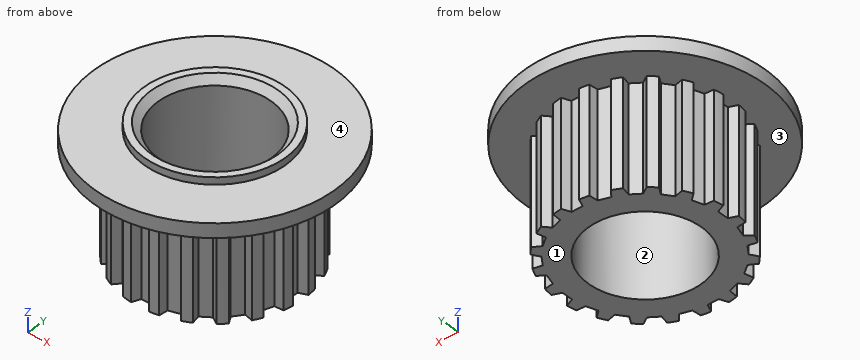
```python
from build123d import *

# Parameters (mm, degrees)
CUT_EXTRUDE1_DEPTH       = 3
CHAMFER1_SIZE            = 0.259911356
CHAMFER1_SIZE2           = 0.226339217
CUT_EXTRUDE2_START       = 1
CUT_EXTRUDE2_2_OUTLINE_W = 16
CUT_EXTRUDE2_2_OUTLINE_H = 4
CUT_EXTRUDE2_2_DEPTH     = 6.45
CUT_EXTRUDE2_START_2     = 7.45
CUT_EXTRUDE2_3_OUTLINE_R = 5
CUT_EXTRUDE2_3_DEPTH     = 7.5


with BuildPart() as part:
    # Sketch1 → Revolve1 (revolve)
    with BuildSketch(Plane.XY.offset(3.725), mode=Mode.PRIVATE) as revolve1_sk:
        Polygon((1.614337285, 9), (0, 9), (0, 5), (0.595828025, 5), (1.614337285, 5.592863599), align=None)
    revolve(revolve1_sk.sketch.rotate(Axis((0, 9, 3.725), (0, -1, 0)), 270), axis=Axis((0, 9, 3.725), (0, -1, 0)))

    # Sketch2 → Cut-Extrude1 (cut)
    with BuildSketch(Plane(origin=(0, 9, 0), x_dir=(-1, 0, 0), z_dir=(0, 1, 0))):
        Polygon((0.877701457, 2.974684409), (1.088643091, 4.109953963), (0.210941634, 4.860269554), (-0.877701457, 4.475315591), (-1.088643091, 3.340046037), (-0.210941634, 2.589730446), align=None)
    extrude(amount=-CUT_EXTRUDE1_DEPTH, mode=Mode.SUBTRACT)

    # Chamfer1
    chamfer1_edges = [part.edges().sort_by_distance(p)[0] for p in [
        (0, 9, 5.339337285),
    ]]
    chamfer1_side = [part.faces().sort_by_distance(p)[0] for p in [
        (0, 9, 5.293676931),
    ]]
    chamfer(chamfer1_edges, length=CHAMFER1_SIZE, length2=CHAMFER1_SIZE2, reference=chamfer1_side[0])

    # Cut-Extrude2 2 outline → Cut-Extrude2 2 (cut)
    with BuildSketch(Plane.XY.offset(CUT_EXTRUDE2_START)):
        with Locations((0, 7)):
            Rectangle(CUT_EXTRUDE2_2_OUTLINE_W, CUT_EXTRUDE2_2_OUTLINE_H)
    extrude(amount=CUT_EXTRUDE2_2_DEPTH, mode=Mode.SUBTRACT)


with BuildPart() as body_2:
    # Cut-Extrude2: read off the stored shape, not the designer's step
    # Cut-Extrude2 outline → Cut-Extrude2 (revolve)
    with BuildSketch(Plane.XZ):
        Polygon((4, 7.45), (5, 7.45), (5, 14.95), (8.5, 14.95), (8.5, 15.95), (5, 15.95), (5, 16.45), (4.5, 16.45), (4, 15.95), align=None)
    revolve(axis=Axis((0, 0, 0), (0, 0, 1)))

    # Cut-Extrude2 3 outline → Cut-Extrude2 3 (add)
    with BuildSketch(Plane.XY.offset(CUT_EXTRUDE2_START_2)):
        with BuildLine():
            Line((1.30065941, -6.077376909), (1.350072562, -5.449523289))
            Line((1.350072562, -5.449523289), (2.110917775, -5.202309694))
            Line((2.110917775, -5.202309694), (2.519936953, -5.681209621))
            ThreePointArc((2.519936953, -5.681209621), (2.821550956, -5.537605548), (3.115013354, -5.37800305))
            Line((3.115013354, -5.37800305), (2.967990615, -4.765609269))
            Line((2.967990615, -4.765609269), (3.615204211, -4.295381068))
            Line((3.615204211, -4.295381068), (4.152192781, -4.624448087))
            ThreePointArc((4.152192781, -4.624448087), (4.394668645, -4.394668645), (4.624448087, -4.152192781))
            Line((4.624448087, -4.152192781), (4.295381068, -3.615204211))
            Line((4.295381068, -3.615204211), (4.765609269, -2.967990615))
            Line((4.765609269, -2.967990615), (5.37800305, -3.115013354))
            ThreePointArc((5.37800305, -3.115013354), (5.537605548, -2.821550956), (5.681209621, -2.519936953))
            Line((5.681209621, -2.519936953), (5.202309694, -2.110917775))
            Line((5.202309694, -2.110917775), (5.449523289, -1.350072562))
            Line((5.449523289, -1.350072562), (6.077376909, -1.30065941))
            ThreePointArc((6.077376909, -1.30065941), (6.138483037, -0.9722402), (6.181854773, -0.641012138))
            Line((6.181854773, -0.641012138), (5.6, -0.4))
            Line((5.6, -0.4), (5.6, 0.4))
            Line((5.6, 0.4), (6.181854773, 0.641012138))
            ThreePointArc((6.181854773, 0.641012138), (6.138483037, 0.9722402), (6.077376909, 1.30065941))
            Line((6.077376909, 1.30065941), (5.449523289, 1.350072562))
            Line((5.449523289, 1.350072562), (5.202309694, 2.110917775))
            Line((5.202309694, 2.110917775), (5.681209621, 2.519936953))
            ThreePointArc((5.681209621, 2.519936953), (5.537605548, 2.821550956), (5.37800305, 3.115013354))
            Line((5.37800305, 3.115013354), (4.765609269, 2.967990615))
            Line((4.765609269, 2.967990615), (4.295381068, 3.615204211))
            Line((4.295381068, 3.615204211), (4.624448087, 4.152192781))
            ThreePointArc((4.624448087, 4.152192781), (4.394668645, 4.394668645), (4.152192781, 4.624448087))
            Line((4.152192781, 4.624448087), (3.615204211, 4.295381068))
            Line((3.615204211, 4.295381068), (2.967990615, 4.765609269))
            Line((2.967990615, 4.765609269), (3.115013354, 5.37800305))
            ThreePointArc((3.115013354, 5.37800305), (2.821550956, 5.537605548), (2.519936953, 5.681209621))
            Line((2.519936953, 5.681209621), (2.110917775, 5.202309694))
            Line((2.110917775, 5.202309694), (1.350072562, 5.449523289))
            Line((1.350072562, 5.449523289), (1.30065941, 6.077376909))
            ThreePointArc((1.30065941, 6.077376909), (0.9722402, 6.138483037), (0.641012138, 6.181854773))
            Line((0.641012138, 6.181854773), (0.4, 5.6))
            Line((0.4, 5.6), (-0.4, 5.6))
            Line((-0.4, 5.6), (-0.641012138, 6.181854773))
            ThreePointArc((-0.641012138, 6.181854773), (-0.9722402, 6.138483037), (-1.30065941, 6.077376909))
            Line((-1.30065941, 6.077376909), (-1.350072562, 5.449523289))
            Line((-1.350072562, 5.449523289), (-2.110917775, 5.202309694))
            Line((-2.110917775, 5.202309694), (-2.519936953, 5.681209621))
            ThreePointArc((-2.519936953, 5.681209621), (-2.821550956, 5.537605548), (-3.115013354, 5.37800305))
            Line((-3.115013354, 5.37800305), (-2.967990615, 4.765609269))
            Line((-2.967990615, 4.765609269), (-3.615204211, 4.295381068))
            Line((-3.615204211, 4.295381068), (-4.152192781, 4.624448087))
            ThreePointArc((-4.152192781, 4.624448087), (-4.394668645, 4.394668645), (-4.624448087, 4.152192781))
            Line((-4.624448087, 4.152192781), (-4.295381068, 3.615204211))
            Line((-4.295381068, 3.615204211), (-4.765609269, 2.967990615))
            Line((-4.765609269, 2.967990615), (-5.37800305, 3.115013354))
            ThreePointArc((-5.37800305, 3.115013354), (-5.537605548, 2.821550956), (-5.681209621, 2.519936953))
            Line((-5.681209621, 2.519936953), (-5.202309694, 2.110917775))
            Line((-5.202309694, 2.110917775), (-5.449523289, 1.350072562))
            Line((-5.449523289, 1.350072562), (-6.077376909, 1.30065941))
            ThreePointArc((-6.077376909, 1.30065941), (-6.138483037, 0.9722402), (-6.181854773, 0.641012138))
            Line((-6.181854773, 0.641012138), (-5.6, 0.4))
            Line((-5.6, 0.4), (-5.6, -0.4))
            Line((-5.6, -0.4), (-6.181854773, -0.641012138))
            ThreePointArc((-6.181854773, -0.641012138), (-6.138483037, -0.9722402), (-6.077376909, -1.30065941))
            Line((-6.077376909, -1.30065941), (-5.449523289, -1.350072562))
            Line((-5.449523289, -1.350072562), (-5.202309694, -2.110917775))
            Line((-5.202309694, -2.110917775), (-5.681209621, -2.519936953))
            ThreePointArc((-5.681209621, -2.519936953), (-5.537605548, -2.821550956), (-5.37800305, -3.115013354))
            Line((-5.37800305, -3.115013354), (-4.765609269, -2.967990615))
            Line((-4.765609269, -2.967990615), (-4.295381068, -3.615204211))
            Line((-4.295381068, -3.615204211), (-4.624448087, -4.152192781))
            ThreePointArc((-4.624448087, -4.152192781), (-4.394668645, -4.394668645), (-4.152192781, -4.624448087))
            Line((-4.152192781, -4.624448087), (-3.615204211, -4.295381068))
            Line((-3.615204211, -4.295381068), (-2.967990615, -4.765609269))
            Line((-2.967990615, -4.765609269), (-3.115013354, -5.37800305))
            ThreePointArc((-3.115013354, -5.37800305), (-2.821550956, -5.537605548), (-2.519936953, -5.681209621))
            Line((-2.519936953, -5.681209621), (-2.110917775, -5.202309694))
            Line((-2.110917775, -5.202309694), (-1.350072562, -5.449523289))
            Line((-1.350072562, -5.449523289), (-1.30065941, -6.077376909))
            ThreePointArc((-1.30065941, -6.077376909), (-0.9722402, -6.138483037), (-0.641012138, -6.181854773))
            Line((-0.641012138, -6.181854773), (-0.4, -5.6))
            Line((-0.4, -5.6), (0.4, -5.6))
            Line((0.4, -5.6), (0.641012138, -6.181854773))
            ThreePointArc((0.641012138, -6.181854773), (0.9722402, -6.138483037), (1.30065941, -6.077376909))
        make_face()
        Circle(CUT_EXTRUDE2_3_OUTLINE_R, mode=Mode.SUBTRACT)
    extrude(amount=CUT_EXTRUDE2_3_DEPTH)


solid = body_2.part
```
Geometry check sheet. Reference: the model listing, model coordinates, mm. Face numbers are marked on the shaded views. A direction names the side the tool comes from. Give positions to 0.01 mm unless a question says otherwise; leave off trailing zeros. Write each loop counter-clockwise with the first axis right and the second up, starting at its lowest first coordinate (ties: lowest second). Pieces come first, ordered by that corner, then holes. Notation, with made-up numbers: (-22, -28.5) -> (0, -28.5) arc R28 cw to (0, -2.5) -> close; hole circle Ø2 at (75, -16). An arc over 180 degrees is marked (long way). Use one line per item in the form item = value.
Item 1: Access from +Z, -Z, +X, -X, +Y, -Y to the whole of each face (thin tool, end or side, straight path). Record for the marked faces 3 and 4.
Results list:
face_3 = -Z
face_4 = +Z
Item 2: Sectioned sample at C-C on y = -7.25. Enter the section's corners in (x, z).
Results list:
outline = (-4.44, 14.95) -> (4.44, 14.95) -> (4.44, 15.95) -> (-4.44, 15.95) -> close
Item 3: Depth check by flat-ended pin: pin 1 Ø3 at (x, y) = (0.5, -1.5) entering from -Z; pin 2 Ø0.9 at (y, z) = (0, 11) entering from +X; pin 3 Ø3 at (x, z) = (-1, 10) entering from -Y; pin 4 Ø1.5 at (y, z) = (1.5, 8.5) entering from +X. Enter the tip coordinate at first touch or a pass-through.
Results list:
pin_1 = through
pin_2 = 5.72
pin_3 = -6.18
pin_4 = 6.17
Item 4: Sectioned sample at A-A on x = 0. Enter the section's corners in (y, z), plus the area to 4 significant figures.
Results list:
outline = (-8.5, 14.95) -> (-5.6, 14.95) -> (-5.6, 7.45) -> (-4, 7.45) -> (-4, 15.95) -> (-4.5, 16.45) -> (-5, 16.45) -> (-5, 15.95) -> (-8.5, 15.95) -> close; (4, 7.45) -> (5.6, 7.45) -> (5.6, 14.95) -> (8.5, 14.95) -> (8.5, 15.95) -> (5, 15.95) -> (5, 16.45) -> (4.5, 16.45) -> (4, 15.95) -> close
area = 33.75 mm2
Item 5: Mould release check, pull along X, two halves, no side actions. Record for the marked faces 1 and 2: released by +X, released by -X, zero draft, split by the parting line, or undercut.
Results list:
face_1 = zero draft
face_2 = undercut
Item 6: Sectioned sample at D-D on y = 7. Enter the section's corners in (x, z).
Results list:
outline = (-4.82, 14.95) -> (4.82, 14.95) -> (4.82, 15.95) -> (-4.82, 15.95) -> close
Item 7: Scan lines: line 1 (Y direction, x = 0, z = 10); line 2 (Y direction, x = -2.5, z = 9.5); line 3 (Z direction, x = 5, y = -2). Record each from-to range of solid material in increasing order.
Results list:
line_1 = -5.6 to -4, 4 to 5.6
line_2 = -5.66 to -3.12, 3.12 to 5.66
line_3 = 7.45 to 15.95
